Design review of the part built by this model. Coordinates are the model's own, in mm. A direction names the side the tool comes from. Coordinates: 2 decimals unless noted, no trailing zeros. Order: outer loops, then holes, each group sorted by start corner. A loop starts at its lowest first (then second) coordinate and runs counter-clockwise, first axis right, second up. Notation, with made-up numbers: (38.25, 31.25) -> (95.25, 31.25) arc R23 ccw to (95.25, 61.25) -> close; hole circle Ø10 at (52.25, 48.5). An arc over 180 degrees is marked (long way). Write item = value, one per line.
```python
from build123d import *

# Parameters (mm, degrees)
F0_W     = 31.75
F0_H     = 15.75
F1_DEPTH = 9.5
F2_W     = 31
F2_H     = 15
F3_DEPTH = 8.5
F5_DEPTH = 2
F6_R     = 2.4
F7_DEPTH = 6.1


with BuildPart() as f1:
    # F0 (on Front) → F1 (new body)
    with BuildSketch(Plane.XZ):
        Rectangle(F0_W, F0_H)
    extrude(amount=F1_DEPTH)

    # F2 (on face) → F3 (cut)
    with BuildSketch(Plane(origin=(0, 0, 0), x_dir=(-1, 0, 0), z_dir=(0, 1, 0))):
        Rectangle(F2_W, F2_H)
    extrude(amount=-F3_DEPTH, mode=Mode.SUBTRACT)

    # F4 (on face) → F5 (join)
    with BuildSketch(Plane.XZ.offset(9.5)):
        with BuildLine():
            ThreePointArc((-1.515, -3.665893), (-3.071941, -1.384458), (-5.763935, -2.002664))
            ThreePointArc((-5.763935, -2.002664), (-4.858059, -5.947328), (-1.515, -3.665893))
        make_face()
        with BuildLine():
            ThreePointArc((-9.145893, -3.965), (-9.351187, -2.98327), (-9.932664, -2.166065))
            ThreePointArc((-9.932664, -2.166065), (-13.8406, -4.94673), (-9.145893, -3.965))
        make_face()
        with BuildLine():
            ThreePointArc((-9.145893, 3.389351), (-13.877328, 4.28241), (-9.796958, 1.726121))
            ThreePointArc((-9.796958, 1.726121), (-9.314458, 2.496292), (-9.145893, 3.389351))
        make_face()
        with BuildLine():
            ThreePointArc((-1.814107, 3.965), (-5.245837, 6.209706), (-5.927336, 2.166065))
            ThreePointArc((-5.927336, 2.166065), (-3.282376, 1.720294), (-1.814107, 3.965))
        make_face()
        with BuildLine():
            ThreePointArc((6.365, 3.665893), (1.730125, 4.540727), (5.727222, 2.036607))
            ThreePointArc((5.727222, 2.036607), (6.199875, 2.79106), (6.365, 3.665893))
        make_face()
        with BuildLine():
            ThreePointArc((13.995893, 3.965), (10.634199, 6.163896), (9.966607, 2.202778))
            ThreePointArc((9.966607, 2.202778), (12.557588, 1.766104), (13.995893, 3.965))
        make_face()
        with BuildLine():
            ThreePointArc((14.295, -3.665893), (12.769833, -1.431018), (10.132778, -2.036607))
            ThreePointArc((10.132778, -2.036607), (11.020167, -5.900769), (14.295, -3.665893))
        make_face()
        with BuildLine():
            ThreePointArc((6.664107, -3.965), (6.463002, -3.003305), (5.893393, -2.202778))
            ThreePointArc((5.893393, -2.202778), (2.065211, -4.926695), (6.664107, -3.965))
        make_face()
    extrude(amount=F5_DEPTH)

    # F6 (on face) → F7 (join)
    with BuildSketch(Plane(origin=(0, -8.5, 0), x_dir=(-1, 0, 0), z_dir=(0, 1, 0))):
        with BuildLine():
            ThreePointArc((0, -3.25), (2.298097, -2.298097), (3.25, 0))
            ThreePointArc((3.25, 0), (2.298097, 2.298097), (0, 3.25))
            ThreePointArc((0, 3.25), (-3.25, 0), (0, -3.25))
        make_face()
        Circle(F6_R, mode=Mode.SUBTRACT)
    extrude(amount=F7_DEPTH)


solid = f1.part
```
(1) We need section C-C (x = 13). Write out the cut boundary in (y, z) (3 decimals).
Report:
outline = (-11.5, -5.796) -> (-9.5, -5.796) -> (-9.5, -7.875) -> (0, -7.875) -> (0, -7.5) -> (-8.5, -7.5) -> (-8.5, 7.5) -> (0, 7.5) -> (0, 7.875) -> (-9.5, 7.875) -> (-9.5, 5.911) -> (-11.5, 5.911) -> (-11.5, 2.019) -> (-9.5, 2.019) -> (-9.5, -1.535) -> (-11.5, -1.535) -> close
(2) We need section A-A (y = -3). Write out the cut boundary in (x, z) (3 decimals).
Report:
outline = (-15.875, -7.875) -> (15.875, -7.875) -> (15.875, 7.875) -> (-15.875, 7.875) -> close; circle Ø6.5 at (0, 0); hole (-15.5, -7.5) -> (15.5, -7.5) -> (15.5, 7.5) -> (-15.5, 7.5) -> close; hole circle Ø4.8 at (0, 0)
(3) We need section B-B (y = -0.75). Write out the cut boundary in (x, z) (3 decimals).
Report:
outline = (-15.875, -7.875) -> (15.875, -7.875) -> (15.875, 7.875) -> (-15.875, 7.875) -> close; hole (-15.5, -7.5) -> (15.5, -7.5) -> (15.5, 7.5) -> (-15.5, 7.5) -> close
(4) For L1, parallel to X at y = -7.75, z = -7 (3 decimals); L2, parallel to Z at x = 3, y = -8.25 (3 decimals); L3, parallel to Z at x = 8.5, y = -6.75 (3 decimals), list the stretches that pass through material, from the lowest coordinate up.
Report:
L1 = -15.875 to -15.5, 15.5 to 15.875
L2 = -7.875 to -7.5, -1.25 to 1.25, 7.5 to 7.875
L3 = -7.875 to -7.5, 7.5 to 7.875
(5) The part is to be moulded in two halves that separate along X. For faces 1 (the flat face through (15.875, -5, 0)), 2 (the flat face through (-12, -11.5, 3)), 3 (the flat face through (0, -4, -7.5)), 4 (the flat face through (0.2, -8.5, 3.4)), say which applies: released by +X, released by -X, zero draft, split by the parting line, or undercut.
Report:
face_1 = released by +X
face_2 = zero draft
face_3 = undercut
face_4 = undercut
(6) Insertion check: pin 1 (2 mm diameter, centred on x = -1.5, y = -10, fed in from +Z) (3 decimals); pin 2 (7.5 mm diameter, centred on x = 4.5, z = 1, fed in from +Y); pin 3 (1 mm diameter, centred on x = 4.5, z = 6, fed in from +Y). Each pin has a flat end and moves straight along its axis. Give the tip position at first contact, or say it passes through.
Report:
pin_1 = 7.875
pin_2 = -2.4
pin_3 = -8.5
(7) For faces 5 (the flat face through (4, -11.5, -4)), 6 (the flat face through (0, -9.5, 0)), 7 (the flat face through (0, -4, 7.5)), list the 3-axis set-ups (+Z, -Z, +X, -X, +Y, -Y) from which the entire face can be reached by the end or side of a thin tool; tool diameter is ignored.
Report:
face_5 = +Z, -Z, +X, -X, -Y
face_6 = -Y
face_7 = +Y
(8) We need section D-D (x = -4.5). Write out the cut boundary in (y, z) (3 decimals), and give its area (3 significant figures).
Report:
outline = (-11.5, -6.057) -> (-9.5, -6.057) -> (-9.5, -7.875) -> (0, -7.875) -> (0, -7.5) -> (-8.5, -7.5) -> (-8.5, 7.5) -> (0, 7.5) -> (0, 7.875) -> (-9.5, 7.875) -> (-9.5, 6.404) -> (-11.5, 6.404) -> (-11.5, 1.526) -> (-9.5, 1.526) -> (-9.5, -1.275) -> (-11.5, -1.275) -> close
area = 41.4 mm²
